Verification items for this drawing (mm, ordinates from the low corner). Give positions to 0.01 mm unless a question says otherwise; leave off trailing zeros. Write each loop counter-clockwise with the first axis right and the second up, starting at its lowest first coordinate (ties: lowest second). Pieces come first, ordered by that corner, then holes. Notation, with made-up numbers: M -23.5,-39.5 L -1.5,-39.5 A22 cw -1.5,-10.5 Z; hole C 66,25 d7. An arc over 180 degrees is marked long. Write each question's results on one line, items separated by ' | '.
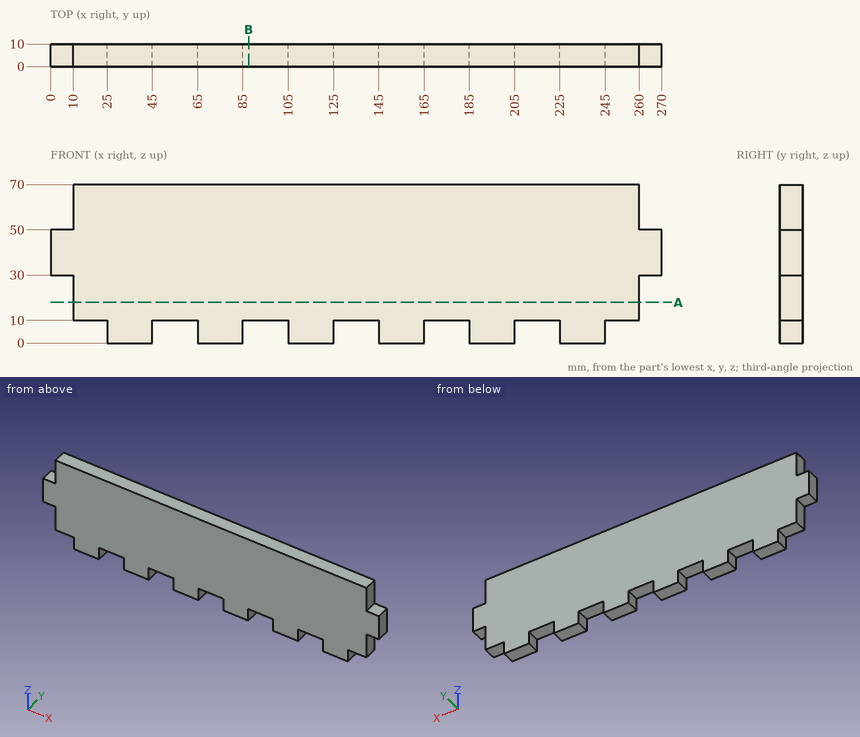
Q1. Material ranges on probe 1 along X at (y, z) = (1.5, 5.5); probe 2 along X at (y, z) = (6.25, 13.5); probe 3 along Z at (x, y) = (53, 4.75), recorded low to high. Write a range as [from, to].
Answer key:
probe 1: x = [25, 45], [65, 85], [105, 125], [145, 165], [185, 205], [225, 245] | probe 2: x = [10, 260] | probe 3: z = [10, 70]
Q2. Depth check by flat-ended pin: P1, Ø5, axis at x = 98.5, y = 4, coming from the -Z side; P2, Ø5, axis at x = 264, y = 3, coming from the -Z side; P3, Ø2, axis at y = 6, z = 18, coming from the +X side; P4, Ø4, axis at x = 28, z = 59.5, coming from the -Y side. Enter the tip coordinate at first touch or a pass-through.
Answer key:
P1: stops at z = 10 | P2: stops at z = 30 | P3: stops at x = 260 | P4: stops at y = 0
Q3. Section check A-A (z = 18). Enter the section's corners in (x, y), then the cut area to 3 significant figures.
Answer key:
outline: M 10,0 L 260,0 L 260,10 L 10,10 Z | area: 2,500 mm2
Q4. Section check B-B (x = 87.5). Enter the section's corners in (y, z), then the cut area to 3 significant figures.
Answer key:
outline: M 0,10 L 10,10 L 10,70 L 0,70 Z | area: 600 mm2
